```python
from build123d import *

# Parameters (mm, degrees)
SKETCH1_W                = 45
SKETCH1_H                = 60
SKETCH1_R                = 1.6
BOSS_EXTRUDE1_DEPTH      = 4.5
CHAMFER1_SIZE            = 1
CUT_EXTRUDE1_DEPTH       = 38.769034936
CUT_EXTRUDE1_DEPTH_BACK  = 38.769034936
SKETCH2_W                = 42.2
SKETCH2_H                = 1.8
BOSS_EXTRUDE2_DEPTH      = 22.5
BOSS_EXTRUDE2_DEPTH_BACK = 22.5
CUT_EXTRUDE2_DEPTH       = 39.684622268
CUT_EXTRUDE2_DEPTH_BACK  = 39.684622268
SKETCH6_W                = 16.662256764
SKETCH6_H                = 27.999999992
SKETCH6_W_2              = 12.602721676
CUT_EXTRUDE3_DEPTH       = 10


with BuildPart() as part:
    # Sketch1 → Boss-Extrude1 (new body)
    with BuildSketch(Plane(origin=(0, 0, 0), x_dir=(1, 0, 0), z_dir=(0, 1, 0))):
        Rectangle(SKETCH1_W, SKETCH1_H)
        with Locations(Location((17.5, 24, 0), (0, 0, 270))):
            Circle(SKETCH1_R, mode=Mode.SUBTRACT)
        with Locations(Location((-17.5, 24, 0), (0, 0, 90))):
            Circle(SKETCH1_R, mode=Mode.SUBTRACT)
        with Locations(Location((-17.5, -24, 0), (0, 0, 270))):
            Circle(SKETCH1_R, mode=Mode.SUBTRACT)
        with Locations(Location((17.5, -24, 0), (0, 0, 90))):
            Circle(SKETCH1_R, mode=Mode.SUBTRACT)
    extrude(amount=BOSS_EXTRUDE1_DEPTH)

    # Chamfer1
    chamfer1_edges = [part.edges().sort_by_distance(p)[0] for p in [
        (0, 0, 30),
        (0, 0, -30),
    ]]
    chamfer(chamfer1_edges, length=CHAMFER1_SIZE)

    # Sketch2 → Cut-Extrude1 (cut, two sides: drawn at the far end of the back side and taken through both)
    with BuildSketch(Plane(origin=(0, 0, 0), x_dir=(0, 0, -1), z_dir=(1, 0, 0)).offset(-CUT_EXTRUDE1_DEPTH_BACK)):
        Rectangle(SKETCH2_W, SKETCH2_H)
    extrude(amount=CUT_EXTRUDE1_DEPTH + CUT_EXTRUDE1_DEPTH_BACK, mode=Mode.SUBTRACT)

    # Sketch4 → Boss-Extrude2 (add, two sides: drawn at the far end of the back side and taken through both)
    with BuildSketch(Plane(origin=(0, 0, 0), x_dir=(0, 0, -1), z_dir=(1, 0, 0)).offset(-BOSS_EXTRUDE2_DEPTH_BACK)):
        Polygon((19, 4.5), (-19, 4.5), (-19, 6.5), (-16, 9.5), (16, 9.5), (19, 6.5), align=None)
    extrude(amount=BOSS_EXTRUDE2_DEPTH + BOSS_EXTRUDE2_DEPTH_BACK)

    # Sketch5 → Cut-Extrude2 (cut, two sides: drawn at the far end of the back side and taken through both)
    with BuildSketch(Plane(origin=(0, 0, 0), x_dir=(0, 0, -1), z_dir=(1, 0, 0)).offset(-CUT_EXTRUDE2_DEPTH_BACK)):
        with BuildLine():
            Line((-0.021267592, 0.9), (0.021267592, 0.9))
            ThreePointArc((0.021267592, 0.9), (0.164249511, 0.960439924), (0.22092951, 1.10495356))
            ThreePointArc((0.22092951, 1.10495356), (3.25, 4.21), (6.27907049, 1.10495356))
            ThreePointArc((6.27907049, 1.10495356), (6.335847144, 0.960340972), (6.479009136, 0.9))
            Line((6.479009136, 0.9), (6.520990864, 0.9))
            ThreePointArc((6.520990864, 0.9), (6.664152856, 0.960340972), (6.72092951, 1.10495356))
            ThreePointArc((6.72092951, 1.10495356), (9.75, 4.21), (12.77907049, 1.10495356))
            ThreePointArc((12.77907049, 1.10495356), (12.835847144, 0.960340972), (12.979009136, 0.9))
            Line((12.979009136, 0.9), (11.734788972, -2.913913916))
            Line((11.734788972, -2.913913916), (-11.720609732, -4.129919609))
            Line((-11.720609732, -4.129919609), (-12.979009136, 0.9))
            ThreePointArc((-12.979009136, 0.9), (-12.835847144, 0.960340972), (-12.77907049, 1.10495356))
            ThreePointArc((-12.77907049, 1.10495356), (-9.75, 4.21), (-6.72092951, 1.10495356))
            ThreePointArc((-6.72092951, 1.10495356), (-6.664152856, 0.960340972), (-6.520990864, 0.9))
            Line((-6.520990864, 0.9), (-6.479009136, 0.9))
            ThreePointArc((-6.479009136, 0.9), (-6.335847144, 0.960340972), (-6.27907049, 1.10495356))
            ThreePointArc((-6.27907049, 1.10495356), (-3.25, 4.21), (-0.22092951, 1.10495356))
            ThreePointArc((-0.22092951, 1.10495356), (-0.164249511, 0.960439924), (-0.021267592, 0.9))
        make_face()
    extrude(amount=CUT_EXTRUDE2_DEPTH + CUT_EXTRUDE2_DEPTH_BACK, mode=Mode.SUBTRACT)

    # Sketch6 → Cut-Extrude3 (cut)
    with BuildSketch(Plane(origin=(0, 9.5, 0), x_dir=(1, 0, 0), z_dir=(0, 1, 0))):
        with Locations((-22.831128379, 0)):
            Rectangle(SKETCH6_W, SKETCH6_H)
        with Locations((20.801360835, 0)):
            Rectangle(SKETCH6_W_2, SKETCH6_H)
    extrude(amount=-CUT_EXTRUDE3_DEPTH, mode=Mode.SUBTRACT)


solid = part.part
```
Input: part model. Units: mm. Frame: model coordinates. A direction names the side the tool comes from. Round coordinates to 2 decimals unless told otherwise and drop trailing zeros. Loops run counter-clockwise (first coordinate to the right, second up) from the corner with the lowest first, then second, coordinate; pieces in that order, holes last. Notation, with made-up numbers: (-10, -1.5) -> (41, -1.5) arc R21 ccw to (41, 27.5) -> close; hole circle Ø11 at (-22, 12.5). An arc over 180 degrees is marked (long way). Write each question's results on one line, items separated by ' | '.
1. Mould query, pull axis X, two halves, no side actions, for faces 6 (the face through (0, 4.5, -25)), 7 (the face through (-14.5, 6, 0)), 8 (the face through (-19.086, 2.218, -23.792)), 9 (the face through (14.5, 6, 0)). Classes: +X half, -X half, draft (parallel to the pull), parting line (faces both ways), or undercut.
Geometry results:
face 6: draft | face 7: -X half | face 8: undercut | face 9: +X half
2. Section C-C (y = 7.5). Return loops of the section in (x, z).
Geometry results:
outline: (-22.5, -18) -> (22.5, -18) -> (22.5, -14) -> (14.5, -14) -> (14.5, 14) -> (22.5, 14) -> (22.5, 18) -> (-22.5, 18) -> (-22.5, 14) -> (-14.5, 14) -> (-14.5, -14) -> (-22.5, -14) -> close
3. Section B-B (z = 24). Return loops of the section in (x, y), and give its area (3 significant figures).
Geometry results:
outline: (-22.5, 0) -> (-19.1, 0) -> (-19.1, 4.5) -> (-22.5, 4.5) -> close; (-15.9, 0) -> (15.9, 0) -> (15.9, 4.5) -> (-15.9, 4.5) -> close; (19.1, 0) -> (22.5, 0) -> (22.5, 4.5) -> (19.1, 4.5) -> close | area: 174 mm2
4. First-contact query: P1, Ø6, axis at x = -16, z = -5.5, coming from the -Y side; P2, Ø1.9, axis at x = -17.5, z = 24, coming from the -Y side; P3, Ø4, axis at x = -17.5, z = -24, coming from the +Y side; P4, Ø2.5, axis at x = -20.5, y = 6, coming from the +Z side. Flat tips, straight axial feed; report the tip coordinate or a pass-through.
Geometry results:
P1: y = 0.9 | P2: through | P3: y = 4.5 | P4: z = 19
5. Section A-A (y = 3.25). State how many separate pieces and enclosed holes the cut face has, and give its area (3 significant figures).
Geometry results:
separate pieces: 5 | enclosed holes: 4 | area: 1,710 mm2
6. Set-up query: faces 1 (the face through (18, 5, -14)), 2 (the face through (0, 6, -19)), 3 (the face through (-0.3, 8, 17.5)), 4 (the face through (-19, 5, -14)), 5 (the face through (0, 0.9, 17)). Return all of +Z, -Z, +X, -X, +Y, -Y with unobstructed straight access to the full face (end or side cutting, diameter ignored); none if empty.
Geometry results:
face 1: +X, +Y, -Y | face 2: -Z, +X, -X, +Y | face 3: +Z, +X, -X, +Y | face 4: -X, +Y, -Y | face 5: +X, -X, -Y
7. Ray query, line 1 (X direction, y = 2.25, z = 24); line 2 (Z direction, x = 17, y = 1.5); line 3 (Z direction, x = -4, y = 1.5). Return the intervals inside material, ascending. Write a range as from..to.
Geometry results:
line 1: -22.5..-19.1, -15.9..15.9, 19.1..22.5 | line 2: -30..-25.52, -22.48..-14, 14..22.48, 25.52..30 | line 3: -30..-12.76, -6.74..-6.26, -0.24..0.24, 6.26..6.74, 12.76..30
